Source: CAD feature listing. Evaluate the final solid. Frame: model axes, mm. A direction names the side the tool comes from. Coordinates: 2 decimals unless noted, no trailing zeros. Order: outer loops, then holes, each group sorted by start corner. A loop starts at its lowest first (then second) coordinate and runs counter-clockwise, first axis right, second up.
```python
from build123d import *

# Parameters (mm, degrees)
F1_DEPTH = 25.4
F2_SIZE  = 1.65099


# Not quite as in the source:
# - a fillet or chamfer is up to 0.001 mm smaller than in the source, because OpenCascade refuses the exact size


with BuildPart() as f1:
    # F0 (on Top) → F1 (new body)
    with BuildSketch(Plane.XY):
        with BuildLine():
            ThreePointArc((24.8022671705, 5.4779141289), (28.575, 25.2007812379), (8.5352328295, 23.9229973153))
            ThreePointArc((8.5352328295, 23.9229973153), (-0.6536534353, 25.3915879217), (-9.754807335, 23.4521584051))
            ThreePointArc((-9.754807335, 23.4521584051), (-27.6224996448, 24.3607548834), (-24.4875679847, 6.7467780603))
            ThreePointArc((-24.4875679847, 6.7467780603), (-0.6536534353, -25.3915879217), (24.8022671705, 5.4779141289))
        make_face()
        with BuildLine():
            ThreePointArc((-20.2845825482, 8.7668303761), (-25.1459996448, 22.1766871761), (-11.2336426791, 19.0296315298))
            ThreePointArc((-11.2336426791, 19.0296315298), (-0.6492677951, 22.0884597772), (10.0965, 19.6566093656))
            ThreePointArc((10.0965, 19.6566093656), (26.0985, 23.0167135306), (20.7645, 7.5602343714))
            ThreePointArc((20.7645, 7.5602343714), (-0.6492677951, -22.0884597772), (-20.2845825482, 8.7668303761))
        make_face(mode=Mode.SUBTRACT)
    extrude(amount=F1_DEPTH)

    # F2 (size 1.651 in the source; OpenCascade refuses exactly that, so slightly less here)
    f2_edges = [f1.edges().sort_by_distance(p)[0] for p in [
        (-0.653653, -25.391588, 0),
        (-0.649268, -22.08846, 0),
        (-25.146, 22.176687, 0),
        (-27.6225, 24.360755, 0),
        (-0.649268, 22.08846, 0),
        (-0.653653, 25.391588, 0),
        (28.575, 25.200781, 0),
        (26.0985, 23.016714, 0),
    ]]
    chamfer(f2_edges, length=F2_SIZE)


solid = f1.part
```
1. Material intervals for line 1 along X through (y, z) = (16.5, 10.25); line 2 along X through (y, z) = (0, 10), sorted ascending.
2. Contact query for flat-ended pins moving along their axis: P1, Ø3, axis at y = -17, z = 18, coming from the +X side; P2, Ø21.5, axis at x = 19.05, y = 16.8, coming from the -Z side; P3, Ø6, axis at x = -21, z = 20, coming from the -Y side; P4, Ø13, axis at x = -19.05, y = 16.8, coming from the -Z side. Output: stop coordinate, or through.
3. Section query B-B, the plane z = 7.5. Output: boundary loops of the cut face in (x, y).
4. Access query for faces 1 (the conical face through (-0.816, 22.37, 1.364)), 2 (the cylindrical face through (-0.523, 25.395, 13.359)), 3 (the cylindrical face through (-0.805, 22.083, 13.359)). Directions: +Z, -Z, +X, -X, +Y, -Y. A direction counts if a zero-diameter tool reaches every point of the face in a straight line with its end or side. Return the directions, or none.
5. Draft query along Y for faces 4 (the conical face through (-0.047, -22.385, 1.364)), 5 (the flat face through (-2, 23, 25.4)), 6 (the conical face through (-0.504, 24.191, 0.447)). Return one class per face: +Y half, -Y half, draft (parallel to the pull), parting line (faces both ways), or undercut.
Answer key:
1. line 1: x = -30.48 to -27.17, 28.44 to 31.75
1. line 2: x = -25.4 to -22.1, 22.1 to 25.4
2. P1: stops at x = 20.12
2. P2: stops at z = 0.3
2. P3: stops at y = -17.92
2. P4: passes through
3. outline: (-24.49, 6.75) arc R25.4 ccw (long way) to (24.8, 5.48) arc R12.7 ccw (long way) to (8.54, 23.92) arc R25.4 ccw to (-9.75, 23.45) arc R11.43 ccw (long way) to start; hole (-20.28, 8.77) arc R22.1 ccw (long way) to (20.76, 7.56) arc R9.4 ccw (long way) to (10.1, 19.66) arc R22.1 ccw to (-11.23, 19.03) arc R8.13 ccw (long way) to start
4. face 1: -Z
4. face 2: +Z, -Z, +Y
4. face 3: +Z, -Z
5. face 4: undercut
5. face 5: draft
5. face 6: +Y half
